Part model, mm, in its own coordinate system. Coordinates: 2 decimals unless noted, no trailing zeros. Write each loop counter-clockwise with the first axis right and the second up, starting at its lowest first coordinate (ties: lowest second). Pieces come first, ordered by that corner, then holes. Notation, with made-up numbers: M -25.5,50 L -7.5,50 A22 ccw -7.5,76 Z; hole C 48,-37.75 d3. An arc over 180 degrees is marked long. Use a Markdown table: item, result. Add a question column.
Q1. Slice it at A-A on x = 0. Write the cut outline in (y, z) (3 decimals), then the cut area to 3 significant figures.
Q2. Slice it at B-B on z = 0. Write the cut outline in (x, y) (3 decimals), then the cut area to 3 significant figures.
Q3. Wall check: L1, parallel to Y at x = 0, z = -48.75 (3 decimals); L2, parallel to Z at x = 24.5, y = 17; L3, parallel to Y at x = -7.5, z = -44.5. Give the ranges that are in metal, low to high. Write a range as from..to.
Q4. Slice it at D-D on y = 10. Write the cut outline in (x, z) (3 decimals).
Q5. Mould opens along Z. For faces 1 (the cylindrical face through (-11.7, 25.04, 52.69)), 2 (the cylindrical face through (-1.24, 34.844, 43.646)), 3 (the cylindrical face through (16.116, 25.756, 30.984)) say: released by +Z, released by -Z, zero draft, split by the parting line, or undercut.
Q6. Pin check, flat tips, straight feed: pin 1 Ø6 at (y, z) = (7, -10) entering from -X; pin 2 Ø6 at (x, y) = (-28.5, 27) entering from -Z; pin 3 Ø2 at (y, z) = (8.5, 42) entering from +X; pin 4 Ø15 at (x, y) = (0, 25.4) entering from -Z. Stop position of each tip, or through.
Q7. Slice it at C-C on y = 30.5. Write the cut outline in (x, z) (3 decimals).
from build123d import *

# Parameters (mm, degrees)
SKETCH1_R               = 53.975
BOSS_EXTRUDE1_DEPTH     = 50.8
SKETCH2_R               = 34.925
CUT_EXTRUDE1_DEPTH      = 51.8
SKETCH4_R               = 9.525
CUT_EXTRUDE3_DEPTH      = 54.975
CUT_EXTRUDE3_DEPTH_BACK = 54.975


with BuildPart() as part:
    # Sketch1 → Boss-Extrude1 (new body)
    with BuildSketch(Plane(origin=(0, 0, 0), x_dir=(1, 0, 0), z_dir=(0, 1, 0))):
        Circle(SKETCH1_R)
    extrude(amount=BOSS_EXTRUDE1_DEPTH)

    # Sketch2 → Cut-Extrude1 (cut, through all)
    with BuildSketch(Plane(origin=(0, 50.8, 0), x_dir=(1, 0, 0), z_dir=(0, 1, 0))):
        Circle(SKETCH2_R)
    extrude(amount=-CUT_EXTRUDE1_DEPTH, mode=Mode.SUBTRACT)

    # Sketch4 → Cut-Extrude3 (cut, two sides)
    with BuildSketch(Plane.XY) as cut_extrude3_sk:
        with Locations((0, 25.4)):
            Circle(SKETCH4_R)
    extrude(amount=CUT_EXTRUDE3_DEPTH, mode=Mode.SUBTRACT)
    extrude(cut_extrude3_sk.sketch, amount=-CUT_EXTRUDE3_DEPTH_BACK, mode=Mode.SUBTRACT)


solid = part.part
Recorded:
| question | item | result |
|---|---|---|
| 1 | outline | M 0,-53.975 L 15.875,-53.975 L 15.875,-34.925 L 0,-34.925 Z; M 0,34.925 L 15.875,34.925 L 15.875,53.975 L 0,53.975 Z; M 34.925,-53.975 L 50.8,-53.975 L 50.8,-34.925 L 34.925,-34.925 Z; M 34.925,34.925 L 50.8,34.925 L 50.8,53.975 L 34.925,53.975 Z |
| 1 | area | 1,210 mm² |
| 2 | outline | M -53.975,0 L -34.925,0 L -34.925,50.8 L -53.975,50.8 Z; M 34.925,0 L 53.975,0 L 53.975,50.8 L 34.925,50.8 Z |
| 2 | area | 1,940 mm² |
| 3 | L1 | 0..15.875, 34.925..50.8 |
| 3 | L2 | -48.09..-24.89, 24.89..48.09 |
| 3 | L3 | 0..19.53, 31.27..50.8 |
| 4 | outline | C 0,0 d107.95; hole C 0,0 d69.85 |
| 5 | face 1 | split by the parting line |
| 5 | face 2 | zero draft |
| 5 | face 3 | undercut |
| 6 | pin 1 | x = -53.52 |
| 6 | pin 2 | z = -47.57 |
| 6 | pin 3 | x = 35.1 |
| 6 | pin 4 | through |
| 7 | outline | M -8.045,-53.372 L -8.045,-33.986 A34.925 cw -8.045,33.986 L -8.045,53.372 A53.975 ccw Z; M 8.045,-53.372 A53.975 ccw 8.045,53.372 L 8.045,33.986 A34.925 cw 8.045,-33.986 Z |
